from build123d import *

# Parameters (mm, degrees)
BOSS_EXTRUDE1_DEPTH = 6
SKETCH3_R           = 1.75
CUT_EXTRUDE1_DEPTH  = 6
SKETCH4_R           = 5.5
SKETCH4_R_2         = 3
BOSS_EXTRUDE2_DEPTH = 24


with BuildPart() as part:
    # Sketch2 → Boss-Extrude1 (new body)
    with BuildSketch(Plane.XY):
        Polygon((0, 6.95), (-6.018876556, 3.475), (-6.018876556, -3.475), (0, -6.95), (6.018876556, -3.475), (6.018876556, 3.475), align=None)
    extrude(amount=BOSS_EXTRUDE1_DEPTH)

    # Sketch3 → Cut-Extrude1 (cut)
    with BuildSketch(Plane.XY.offset(6)):
        Circle(SKETCH3_R)
    extrude(amount=-CUT_EXTRUDE1_DEPTH, mode=Mode.SUBTRACT)

    # Sketch4 → Boss-Extrude2 (add)
    with BuildSketch(Plane(origin=(0, 0, 0), x_dir=(-1, 0, 0), z_dir=(0, 0, -1))):
        Circle(SKETCH4_R)
        Circle(SKETCH4_R_2, mode=Mode.SUBTRACT)
    extrude(amount=BOSS_EXTRUDE2_DEPTH)


solid = part.part
The listing builds one solid part. Answer for the finished solid, in the listing's coordinates (mm). A direction names the side the tool comes from. Round coordinates to 2 decimals unless told otherwise and drop trailing zeros. Order: outer loops, then holes, each group sorted by start corner. A loop starts at its lowest first (then second) coordinate and runs counter-clockwise, first axis right, second up. Notation, with made-up numbers: M 1,41 L 52,41 A21 cw 52,47 Z; hole C 85,54.25 d3. An arc over 180 degrees is marked long. Answer in a Markdown table with one row per item. Add a question column.
1) The part is cut by section D-D on x = -4. Determine the outline of the cut face in (y, z).
2) Determine the mould class of faces 3 (the face through (1.617, -0.67, 3.042)), 4 (the face through (1.19, -5.37, -11.83)), 5 (the face through (-3.05, -5.19, 2.96)) for opening direction X: pulls with the +X half, pulls with the -X half, needs draft (parallel to the pull), parting line crosses it, or undercut.
3) The part is cut by section C-C on x = 1. Determine the outline of the cut face in (y, z), plus the area to 3 significant figures.
4) The part is cut by section B-B on y = 0. Determine the outline of the cut face in (x, z).
5) Flat-ended cylindrical pins translate along their axes: pin 1 Ø2 at (x, z) = (-2.5, 0.5) entering from +Y; pin 2 Ø1 at (x, z) = (2, 1) entering from -Y; pin 3 Ø5 at (y, z) = (-5, -17.5) entering from +X. Find the tip coordinate at first contact, or state that the pin passes through.
6) The part is cut by section A-A on z = 1.5. Determine the outline of the cut face in (x, y) (3 decimals).
7) Consider line 1 along Y through (x, z) = (0, -15.25); line 2 along Z through (x, y) = (-0.75, -5.75); line 3 along Y through (x, z) = (-0.75, -8.5). Determine where each line is inside the solid, lowest interval first. Write a range as from..to.
8) Which of the six approach directions +Z, -Z, +X, -X, +Y, -Y give full straight-line access (tool end or side, diameter ignored) to faces 1 (the face through (3, 0, -12)), 2 (the face through (6.019, 0, 3))?
Findings below:
| question | item | result |
|---|---|---|
| 1 | outline | M -4.64,0 L -3.77,0 L -3.77,-24 L 3.77,-24 L 3.77,0 L 4.64,0 L 4.64,6 L -4.64,6 Z |
| 2 | face 3 | undercut |
| 2 | face 4 | parting line crosses it |
| 2 | face 5 | pulls with the -X half |
| 3 | outline | M -6.37,0 L -5.41,0 L -5.41,-24 L -2.83,-24 L -2.83,0 L -1.44,0 L -1.44,6 L -6.37,6 Z; M 1.44,0 L 2.83,0 L 2.83,-24 L 5.41,-24 L 5.41,0 L 6.37,0 L 6.37,6 L 1.44,6 Z |
| 3 | area | 183 mm² |
| 4 | outline | M -6.02,0 L -5.5,0 L -5.5,-24 L -3,-24 L -3,0 L -1.75,0 L -1.75,6 L -6.02,6 Z; M 1.75,0 L 3,0 L 3,-24 L 5.5,-24 L 5.5,0 L 6.02,0 L 6.02,6 L 1.75,6 Z |
| 5 | pin 1 | stops at y = 6.08 |
| 5 | pin 2 | stops at y = -6.08 |
| 5 | pin 3 | stops at x = 4.9 |
| 6 | outline | M -6.019,-3.475 L 0,-6.95 L 6.019,-3.475 L 6.019,3.475 L 0,6.95 L -6.019,3.475 Z; hole C 0,0 d3.5 |
| 7 | line 1 | y = -5.5..-3, 3..5.5 |
| 7 | line 2 | z = 0..6 |
| 7 | line 3 | y = -5.45..-2.9, 2.9..5.45 |
| 8 | face 1 | -Z |
| 8 | face 2 | +Z, -Z, +X, +Y, -Y |
